Autodesk Inventor part; units mm, degrees
ref_plane "Work Plane1" through (30.1625, 0, 0) normal (0, 0, -1) x (1, 0, 0)
ref_plane "YZ Plane" through (0, 0, 0) normal (1, 0, 0) x (0, 1, 0)
ref_plane "XZ Plane" through (0, 0, 0) normal (0, 1, 0) x (-1, 0, 0)
sketch "Sketch1" plane through (0, 0, 0) normal (0, 0, 1) x (1, 0, 0)
  line L0 (-3.3, 0) -> (10, 0)
  line L1 (10, 0) -> (10, 2.5)
  line L2 (10, 2.5) -> (1.6, 2.5)
  line L3 (1.6, 2.5) -> (1.1091, 2.2547)
  line L4 (1.1091, 2.2547) -> (0, 2.2547)
  line L5 (0, 2.2547) -> (0, 4.25)
  line L6 (-5.96, 0) -> (12.66, 0)
  line L7 (0, -0.85) -> (0, 5.1)
  line L8 (-3.3, 0) -> (-3.3, 3.9613)
  line L9 (0, 4.25) -> (-3.3, 3.9613)
  line L10 (1.6, 2.5) -> (0, 2.5) construction
  dimension "d0" = 10
  dimension "d1" = 8.4
  dimension "d2" = 0.4909
  dimension "d3" = 3.3
  dimension "d4" = 5
  dimension "d5" = 4.5095
  dimension "d9" = 8.5
  dimension "d10" = 5
revolve "Body" add sketch "Sketch1" angle 360 about axis through (-3.3, 0, 0) along (1, 0, 0)
sketch "Sketch2" plane through (-3.3, 0, 0) normal (-1, 0, 0) x (0, 0, 1)
  circle A0 centre (0, 0) radius 4.25
  line L0 (0, 0) -> (0, 3.9613)
  line L1 (-4.25, 0.6) -> (4.25, 0.6)
  line L2 (4.25, 0.6) -> (4.25, -0.6)
  line L3 (4.25, -0.6) -> (-4.25, -0.6)
  line L4 (-4.25, -0.6) -> (-4.25, 0.6)
  line L5 (-4.25, 0) -> (4.25, 0) construction
  line L6 (0, 0.6) -> (0, -0.6) construction
  point P0 (0, 0)
  dimension "d11" = 1.2
  dimension "d12" = 8.5
fillet "Fillet1" radius 0.2 1 edges at (-3.3, -3.9613, 0)
extrude "Slot" cut sketch "Sketch2" against normal blind 1.3 contours A0 L3 L1 | L2 L3 A0 | A0 L1 L2 | A0 L4 L1 | L3 L4 A0
thread "Thread"
chamfer "Chamfer1" distance 0.4908 distance2 0.4909 1 edges at (10, -2.5, 0) measured on face at (10, 0.6684, -0.7339)
ref_plane "Work Plane1" through (30.1625, 0, 0) normal (0, 0, -1) x (1, 0, 0)
equation "\"d11\" = SBR"
equation "\"d12\" = KOD"
equation "\"d19\" = STI"
equation "\"d14\" = RR"
equation "\"d15\" = GEL"
equation "\"d17\" = -0.5 * SPD + 0.5 * GD"
equation "\"d0\" = NLG"
equation "\"d1\" = GEL"
equation "\"d3\" = KOH"
equation "\"d4\" = GD"
equation "\"d5\" = BDM"
equation "\"d9\" = KOD"
equation "\"d10\" = KEWI"
equation "\"GD\" = NND"
equation "\"NLG\" = 10"
equation "\"GEL\" = 8.4"
equation "\"KOD\" = 8.5"
equation "\"KOH\" = 3.3"
equation "\"GAL\" = 0.61345 * PTC"
equation "\"SPD\" = NND - 1.2269 * PTC"
equation "\"BDM\" = 4.5095"
equation "\"GUL\" = 0.61345 * PTC"
equation "\"RR\" = 0.2"
equation "\"SBR\" = 1.2"
equation "\"STI\" = 1.3"
equation "\"KEWI\" = 5deg"
equation "\"PTC\" = 0.8"
equation "\"THREADDIA\" = 5"
equation "\"TOA\" = 30deg"
equation "\"NND\" = 5"
equation "\"GD1\" = THREADDIA - 1.2269 * PTC"
properties part number "ISO 1207 - M5 x 10" material "X105CrMo17"
Verification items for the finished model (mm, model axes). A direction names the side the tool comes from. Coordinates: 2 decimals unless noted, no trailing zeros. Loops run counter-clockwise (first coordinate to the right, second up) from the corner with the lowest first, then second, coordinate; pieces in that order, holes last. Notation, with made-up numbers: (55.25, 6) -> (67.25, 6) arc R25 ccw to (67.25, 40) -> close; hole circle Ø1 at (63, 9). An arc over 180 degrees is marked (long way). Write each question's results on one line, items separated by ' | '.
Item 1: Tool access check on faces 5 (the face through (-3.3, 2, 0)), 6 (the face through (-2, 0, 0)). Record the directions out of +Z, -Z, +X, -X, +Y, -Y that give a thin tool (end or side, any length) a straight path to the whole face; none if there is none.
Found:
face 5: +Z, -Z, -X, +Y, -Y | face 6: +Z, -Z, -X
Item 2: Material ranges on L1, parallel to X at y = -0.5, z = -3.25; L2, parallel to X at y = 1, z = -3.5; L3, parallel to X at y = 2.25, z = 0.75, recorded low to high.
Found:
L1: x = -2 to 0 | L2: x = -3.3 to 0 | L3: x = -3.3 to 0, 1.34 to 9.64
Item 3: Section check A-A, the plane y = 0. Enter the section's corners in (x, z), plus the area to 3 significant figures.
Found:
outline: (-2, -4.08) -> (0, -4.25) -> (0, -2.25) -> (1.11, -2.25) -> (1.6, -2.5) -> (9.51, -2.5) -> (10, -2.01) -> (10, 2.01) -> (9.51, 2.5) -> (1.6, 2.5) -> (1.11, 2.25) -> (0, 2.25) -> (0, 4.25) -> (-2, 4.08) -> close | area: 65.7 mm2
Item 4: Section check C-C, the plane x = 7. Enter the section's corners in (y, z), plus the area to 3 significant figures.
Found:
outline: circle Ø5 at (0, 0) | area: 19.6 mm2
Item 5: Gauge pin test, flat ends, axial feed: pin 1 (1.5 mm diameter, centred on x = 7.5, z = -1.5, fed in from +Y); pin 2 (2 mm diameter, centred on x = -1, y = -1, fed in from -Z); pin 3 (1 mm diameter, centred on x = -2.5, z = -1, fed in from -Y). Record the tip position at first contact, or that the pin passes through.
Found:
pin 1: stops at y = 2.38 | pin 2: stops at z = -4.21 | pin 3: stops at y = -4.01
Item 6: Mould release check, pull along X, two halves, no side actions. Record for faces 1 (the face through (10, 0, 0)), 2 (the face through (5.5, -0.54, 2.44)), 3 (the face through (-3.3, -2, 0)), 4 (the face through (0.55, -1.79, 1.37)): +X half, -X half, draft (parallel to the pull), parting line (faces both ways), or undercut.
Found:
face 1: +X half | face 2: draft | face 3: -X half | face 4: undercut
Item 7: Section check B-B, the plane z = 0. Enter the section's corners in (x, y).
Found:
outline: (-3.3, -3.78) arc R0.2 ccw to (-3.12, -3.98) -> (0, -4.25) -> (0, -2.25) -> (1.11, -2.25) -> (1.6, -2.5) -> (9.51, -2.5) -> (10, -2.01) -> (10, 2.01) -> (9.51, 2.5) -> (1.6, 2.5) -> (1.11, 2.25) -> (0, 2.25) -> (0, 4.25) -> (-3.12, 3.98) arc R0.2 ccw to (-3.3, 3.78) -> (-3.3, 0.6) -> (-2, 0.6) -> (-2, -0.6) -> (-3.3, -0.6) -> close
